Geometry check sheet. Reference: the model listing, model coordinates, mm. Face numbers are marked on the shaded views. A direction names the side the tool comes from. Give positions to 0.01 mm unless a question says otherwise; leave off trailing zeros. Write each loop counter-clockwise with the first axis right and the second up, starting at its lowest first coordinate (ties: lowest second). Pieces come first, ordered by that corner, then holes. Notation, with made-up numbers: M 76,-23 L 98,-23 A9 cw 98,-9 Z; hole C 47,-23 d8. An arc over 180 degrees is marked long. Write each question's results on one line, items separated by ' | '.
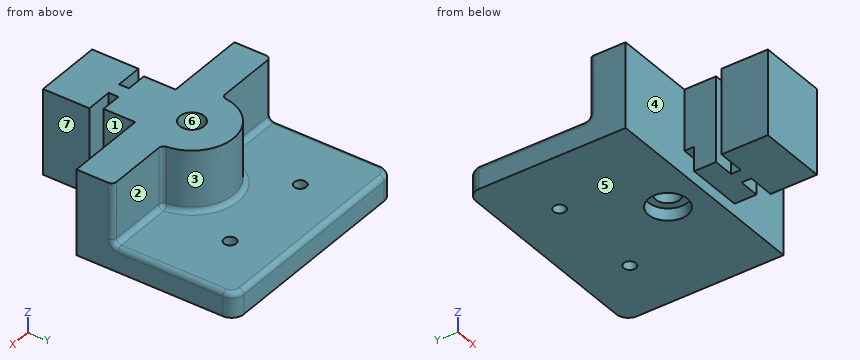
```python
from build123d import *

# Parameters (mm, degrees)
SKETCH_2_W          = 90
SKETCH_2_H          = 101
EXTRUDE_1_DEPTH     = 35
CUT_EXTRUDE_START   = 10
CUT_EXTRUDE_1_DEPTH = 67.491829629
SKETCH_8_R          = 5
CUT_EXTRUDE_3_DEPTH = 77.491829629
SKETCH_9_W          = 23
SKETCH_9_H          = 4
CUT_EXTRUDE_4_DEPTH = 10
HOLE_WIZARD_M5_1_D  = 5
SKETCH_12_R         = 8
CUT_EXTRUDE_5_DEPTH = 5
FILLET_3_R          = 5
FILLET_4_R          = 2


with BuildPart() as part:
    # 草图2 → 凸台-拉伸1 (new body)
    with BuildSketch(Plane.XY):
        with Locations((0, -0.5)):
            Rectangle(SKETCH_2_W, SKETCH_2_H)
    extrude(amount=EXTRUDE_1_DEPTH)

    # 草图3 → 切除-拉伸1 (cut, through all)
    with BuildSketch(Plane.XY.offset(CUT_EXTRUDE_START)):
        with BuildLine():
            Line((45, 50), (-45, 50))
            Line((-45, 50), (-45, 0))
            Line((-45, 0), (-17, 0))
            ThreePointArc((-17, 0), (0, 17), (17, 0))
            Line((17, 0), (45, 0))
            Line((45, 0), (45, 50))
        make_face()
    extrude(amount=CUT_EXTRUDE_1_DEPTH, mode=Mode.SUBTRACT)

    # 草图8 → 切除-拉伸3 (cut, through all)
    with BuildSketch(Plane.XY.offset(35)):
        Circle(SKETCH_8_R)
        Polygon((-45, -15), (-11.5, -15), (-11.5, -28), (-3, -28), (-3, -32), (-14, -32), (-14, -51), (-45, -51), align=None)
        Polygon((45, -51), (45, -15), (11.5, -15), (11.5, -28), (3, -28), (3, -32), (14, -32), (14, -51), align=None)
    extrude(amount=-CUT_EXTRUDE_3_DEPTH, mode=Mode.SUBTRACT)

    # 草图9 → 切除-拉伸4 (cut)
    with BuildSketch(Plane(origin=(0, 0, 0), x_dir=(-1, 0, 0), z_dir=(0, 0, -1))):
        with Locations((0, -17)):
            Rectangle(SKETCH_9_W, SKETCH_9_H)
    extrude(amount=-CUT_EXTRUDE_4_DEPTH, mode=Mode.SUBTRACT)

    # M5 螺纹孔1 (through all)
    with Locations(Plane.XY.offset(10)):
        with Locations((-20, 30), (20, 30)):
            Hole(HOLE_WIZARD_M5_1_D / 2)

    # 草图12 → 切除-拉伸5 (cut)
    with BuildSketch(Plane(origin=(0, 0, 0), x_dir=(-1, 0, 0), z_dir=(0, 0, -1))):
        Circle(SKETCH_12_R)
    extrude(amount=-CUT_EXTRUDE_5_DEPTH, mode=Mode.SUBTRACT)

    # 圆角3
    fillet_3_edges = [part.edges().sort_by_distance(p)[0] for p in [
        (-45, 50, 5),
        (45, 50, 5),
    ]]
    fillet(fillet_3_edges, radius=FILLET_3_R)

    # 圆角4
    fillet_4_edges = [part.edges().sort_by_distance(p)[0] for p in [
        (0, 50, 10),
        (-45, 22.5, 10),
        (-43.535533906, 48.535533906, 10),
        (43.535533906, 48.535533906, 10),
        (45, 22.5, 10),
        (45, 0, 22.5),
        (-31, 0, 10),
        (-45, 0, 22.5),
        (0, 17, 10),
        (-17, 0, 22.5),
        (31, 0, 10),
        (17, 0, 22.5),
    ]]
    fillet(fillet_4_edges, radius=FILLET_4_R)


solid = part.part
```
Q1. Material ranges on probe 1 along Y at (x, z) = (8, 7.5); probe 2 along X at (y, z) = (32, 9); probe 3 along Y at (x, z) = (-20, 7.75), recorded low to high. Write a range as [from, to].
Answer key:
probe 1: y = [-51, -32], [-28, -19], [-15, 50] | probe 2: x = [-44.73, -21.5], [-18.5, 18.5], [21.5, 44.73] | probe 3: y = [-15, 27.5], [32.5, 50]
Q2. Section check A-A (y = 30). Enter the section's corners in (x, z).
Answer key:
outline: M -45,0 L -22.5,0 L -22.5,10 L -43,10 A2 ccw -45,8 Z; M -17.5,0 L 17.5,0 L 17.5,10 L -17.5,10 Z; M 22.5,0 L 45,0 L 45,8 A2 ccw 43,10 L 22.5,10 Z
Q3. Section check D-D (z = 29.5). Enter the section's corners in (x, y), then the cut area to 3 significant figures.
Answer key:
outline: M -45,-15 L -11.5,-15 L -11.5,-28 L -3,-28 L -3,-32 L -14,-32 L -14,-51 L 14,-51 L 14,-32 L 3,-32 L 3,-28 L 11.5,-28 L 11.5,-15 L 45,-15 L 45,-2 A2 ccw 43,0 L 18.89,0 A2 cw 16.91,1.79 A17 ccw -16.91,1.79 A2 cw -18.89,0 L -43,0 A2 ccw -45,-2 Z; hole C 0,0 d10 | area: 2,580 mm2
Q4. Depth check by flat-ended pin: P1, Ø10, axis at x = 3, y = 35.5, coming from the +Z side; P2, Ø10.5, axis at y = -23, z = 10.5, coming from the -X side; P3, Ø3, axis at x = 13.5, y = -30, coming from the -Z side; P4, Ø1.2, axis at y = -30, z = 25.5, coming from the -X side. Enter the tip coordinate at first touch or a pass-through.
Answer key:
P1: stops at z = 10 | P2: stops at x = -11.5 | P3: passes through | P4: stops at x = -3
Q5. Section check C-C (x = -36). Enter the section's corners in (y, z).
Answer key:
outline: M -15,0 L 50,0 L 50,8 A2 ccw 48,10 L 2,10 A2 cw 0,12 L 0,35 L -15,35 Z
Q6. Release check for a two-part mould opening along X. For the marked faces 5, 6 and 7 record: released by +X, released by -X, zero draft, split by the parting line, or undercut.
Answer key:
face 5: zero draft | face 6: undercut | face 7: released by +X
Q7. Access from +Z, -Z, +X, -X, +Y, -Y to the whole of each face (thin tool, end or side, straight path). Record for the marked faces 1, 2, 3 and 4.
Answer key:
face 1: +Z, -Z, +X | face 2: +Z, +X, +Y | face 3: +Z, +Y | face 4: -Z
Q8. Section check B-B (z = 2.5). Enter the section's corners in (x, y), then the cut area to 3 significant figures.
Answer key:
outline: M -45,-15 L 45,-15 L 45,45 A5 ccw 40,50 L -40,50 A5 ccw -45,45 Z; M -14,-51 L 14,-51 L 14,-32 L 3,-32 L 3,-28 L 11.5,-28 L 11.5,-19 L -11.5,-19 L -11.5,-28 L -3,-28 L -3,-32 L -14,-32 Z; hole C -20,30 d5; hole C 0,0 d16; hole C 20,30 d5 | area: 6,360 mm2
